Check sheet for the drawn part. Datum: minimum x, y, z corner. Units: mm. Give positions to 0.01 mm unless a question says otherwise; leave off trailing zeros. Loops run counter-clockwise (first coordinate to the right, second up) from the corner with the lowest first, then second, coordinate; pieces in that order, holes last. Notation, with made-up numbers: M 24.25,-9.75 L 59.25,-9.75 A19 ccw 59.25,15.25 Z; hole C 34,49.5 d10. An arc over 180 degrees is marked long. Write each question's results on one line, items separated by ' | '. Start each with the question number.
1. Sectioned sample at D-D on x = 35. Record the cut outline in (y, z), and give its area (3 significant figures).
2. Sectioned sample at B-B on y = 5. Record the cut outline in (x, z), and give its area (3 significant figures).
3. Sectioned sample at A-A on z = 25. Record the cut outline in (x, y), and give its area (3 significant figures).
4. Draft check along Z on the marked faces 1, 2 and 3. Enter one of: pulls with the +Z half, pulls with the -Z half, needs draft (parallel to the pull), parting line crosses it, or undercut.
5. Go/stop test with flat-tipped pins: pin 1 (9 mm diameter, centred on x = 57.75, z = 25, fed in from -Y); pin 2 (4 mm diameter, centred on x = 35, y = 5, fed in from +Z). Record where each tip stops, or that it passes through.
6. Sectioned sample at C-C on x = 58. Record the cut outline in (y, z), and give its area (3 significant figures).
7. Material ranges on line 1 along Y through (x, z) = (35, 66.5); line 2 along X through (y, z) = (35.5, 27); line 3 along X through (y, z) = (14, 21), recorded low to high.
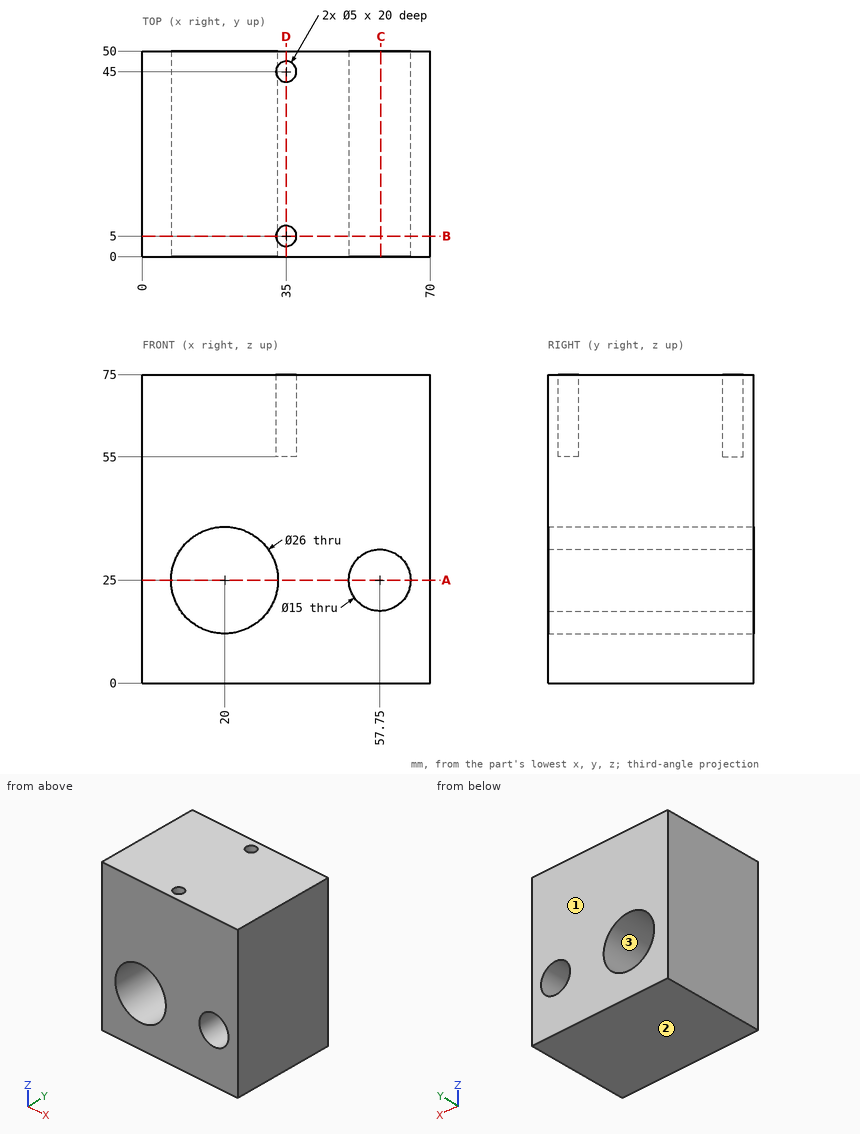
Output values:
1) outline: M 0,0 L 50,0 L 50,75 L 47.5,75 L 47.5,55 L 42.5,55 L 42.5,75 L 7.5,75 L 7.5,55 L 2.5,55 L 2.5,75 L 0,75 Z | area: 3,550 mm2
2) outline: M 0,0 L 70,0 L 70,75 L 37.5,75 L 37.5,55 L 32.5,55 L 32.5,75 L 0,75 Z; hole C 20,25 d26; hole C 57.75,25 d15 | area: 4,440 mm2
3) outline: M 0,0 L 7,0 L 7,50 L 0,50 Z; M 33,0 L 50.25,0 L 50.25,50 L 33,50 Z; M 65.25,0 L 70,0 L 70,50 L 65.25,50 Z | area: 1,450 mm2
4) face 1: needs draft | face 2: pulls with the -Z half | face 3: undercut
5) pin 1: through | pin 2: z = 55
6) outline: M 0,0 L 50,0 L 50,17.5 L 0,17.5 Z; M 0,32.5 L 50,32.5 L 50,75 L 0,75 Z | area: 3,000 mm2
7) line 1: 0 to 2.5, 7.5 to 42.5, 47.5 to 50 | line 2: 0 to 7.15, 32.85 to 50.52, 64.98 to 70 | line 3: 0 to 7.63, 32.37 to 51.41, 64.09 to 70
